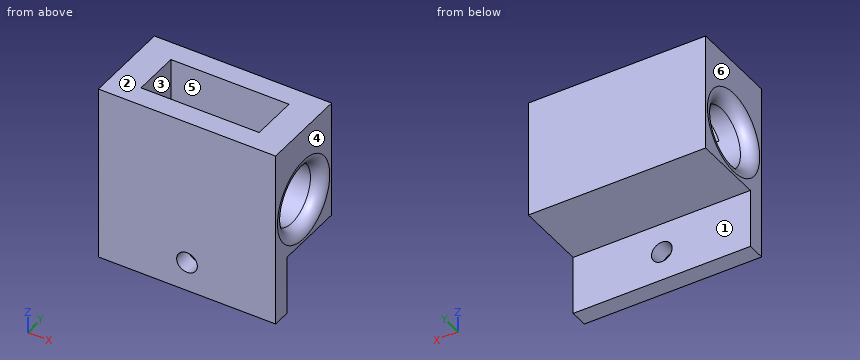
Autodesk Inventor part; units mm, degrees
ref_plane "YZ Plane" through (0, 0, 0) normal (1, 0, 0) x (0, 1, 0)
ref_plane "XZ Plane" through (0, 0, 0) normal (0, 1, 0) x (-1, 0, 0)
ref_plane "XY Plane" through (0, 0, 0) normal (0, 0, 1) x (1, 0, 0)
sketch "Esquisse1" plane through (0, 0, 0) normal (1, 0, 0) x (0, 1, 0)
  circle A0 centre (0, 0) radius 5
  line L0 (7.5, 7.5) -> (-7.5, 7.5)
  line L1 (-7.5, 7.5) -> (-7.5, -7.5)
  line L2 (-7.5, -7.5) -> (7.5, -7.5)
  line L3 (7.5, -7.5) -> (7.5, 7.5)
  line L4 (7.5, 7.5) -> (-7.5, -7.5)
  line L5 (-7.5, 7.5) -> (7.5, -7.5)
  point P0 (0, 0)
  dimension "d0" = 10
  dimension "d1" = 15
  dimension "d2" = 15
extrude "Extrusion1" add sketch "Esquisse1" along normal blind 30 contours A0 L4 L3 L5 | A0 L5 L0 L4 | L5 L2 L4 A0 | A0 L4 L1 L5
sketch "Esquisse6" plane through (0, -7.5, 7.5) normal (0, 0, 1) x (1, 0, 0)
  line L0 (0, 7.5) -> (30, 7.5)
  line L1 (30, 15) -> (30, 0)
  line L2 (5, 11.5) -> (25, 11.5)
  line L3 (25, 11.5) -> (25, 7.5)
  line L4 (25, 7.5) -> (5, 7.5)
  line L5 (5, 7.5) -> (5, 11.5)
  line L6 (0, 15) -> (0, 0)
  line L7 (0, 11.5) -> (5, 11.5)
  line L8 (5, 3.5) -> (25, 3.5)
  line L9 (25, 3.5) -> (25, 7.5)
  line L10 (5, 7.5) -> (5, 3.5)
  dimension "d14" = 4
  dimension "d15" = 5
  dimension "d16" = 20
extrude "Extrusion5" cut sketch "Esquisse6" against normal blind 5 contours L5 L2 L3 L0 | L0 L9 L8 L10
sketch "Esquisse8" plane through (0, -7.5, 7.5) normal (0, 0, 1) x (1, 0, 0)
  line L0 (5, 11.5) -> (25, 11.5)
  line L1 (25, 3.5) -> (5, 3.5)
  line L2 (5, 11.5) -> (25, 11.5)
  line L3 (25, 11.5) -> (25, 3.5)
  line L4 (25, 3.5) -> (5, 3.5)
  line L5 (5, 3.5) -> (5, 11.5)
  line L6 (0, 15) -> (30, 15)
  line L7 (30, 15) -> (30, 0)
  line L8 (0, 15) -> (30, 15)
  line L9 (30, 15) -> (30, 0)
  line L10 (30, 0) -> (0, 0)
  line L11 (0, 0) -> (0, 15)
  point P0 (0, 7.5)
extrude "Extrusion6" add sketch "Esquisse8" along normal blind 5
sketch "Esquisse9" plane through (0, -7.5, -7.5) normal (0, 0, -1) x (-1, 0, 0)
  line L0 (0, 0) -> (-30, 0)
  line L1 (-30, 0) -> (0, 0)
  line L2 (0, 0) -> (0, 3)
  line L3 (0, 3) -> (-30, 3)
  line L4 (-30, 3) -> (-30, 0)
  point P0 (0, 7.5)
extrude "Extrusion7" add sketch "Esquisse9" along normal blind 10
sketch "Esquisse10" plane through (0, -4.5, -7.5) normal (0, 1, 0) x (1, 0, 0)
  circle A0 centre (15, 5) radius 1.75
  line L0 (0, 10) -> (30, 10)
  line L1 (30, 0) -> (30, 10)
  point P0 (0, -7.5)
  dimension "d23" = 3.5
  dimension "d24" = 5
  dimension "d25" = 15
extrude "Extrusion8" cut sketch "Esquisse10" against normal blind 10
fillet "Congé2" radius 2 2 edges at (0, -5, 0) (30, -5, 0)
properties part number "Pièce1_Impression 3D"
Input: part model. Units: mm. Frame: model coordinates. Face numbers are marked on the shaded views. A direction names the side the tool comes from. Coordinates: 2 decimals unless noted, no trailing zeros. Order: outer loops, then holes, each group sorted by start corner. A loop starts at its lowest first (then second) coordinate and runs counter-clockwise, first axis right, second up. Notation, with made-up numbers: M 45,-27 L 80,-27 A22 ccw 80,-11 Z; hole C 51.25,8.25 d2. An arc over 180 degrees is marked long. Answer in a Markdown table with one row per item.
(1) Section query D-D, the plane x = 15. Output: boundary loops of the cut face in (y, z), plus the area to 3 significant figures.
Numbers:
| item | result |
|---|---|
| outline | M -7.5,-17.5 L -4.5,-17.5 L -4.5,-14.25 L -7.5,-14.25 Z; M -7.5,-10.75 L -4.5,-10.75 L -4.5,-7.5 L 7.5,-7.5 L 7.5,12.5 L 4,12.5 L 4,3 A5 cw long -4,3 L -4,12.5 L -7.5,12.5 Z |
| area | 176 mm^2 |
(2) Draft query along X for the marked faces 4, 5 and 6. Return one class per face: pulls with the +X half, pulls with the -X half, needs draft (parallel to the pull), parting line crosses it, or undercut.
Numbers:
| item | result |
|---|---|
| face 4 | pulls with the +X half |
| face 5 | undercut |
| face 6 | pulls with the -X half |
(3) Contact query for flat-ended pins moving along their axis: pin 1 Ø5 at (x, z) = (15.5, -10.5) entering from +Y; pin 2 Ø5 at (y, z) = (-3, 2.5) entering from -X; pin 3 Ø1.5 at (x, y) = (6.5, 5.5) entering from -Z. Output: stop coordinate, or through.
Numbers:
| item | result |
|---|---|
| pin 1 | stops at y = -4.5 |
| pin 2 | stops at x = 0.09 |
| pin 3 | stops at z = -7.5 |
(4) Section query A-A, the plane z = -12.5. Output: boundary loops of the cut face in (x, y), plus the area to 3 significant figures.
Numbers:
| item | result |
|---|---|
| outline | M 0,-7.5 L 13.25,-7.5 L 13.25,-4.5 L 0,-4.5 Z; M 16.75,-7.5 L 30,-7.5 L 30,-4.5 L 16.75,-4.5 Z |
| area | 79.5 mm^2 |
(5) Material intervals for line 1 (Z direction, x = 15, y = -5.9); line 2 (Y direction, x = 16, z = 0); line 3 (X direction, y = 1.75, z = 10.5), sorted ascending. Write a range as [from, to].
Numbers:
| item | result |
|---|---|
| line 1 | z = [-17.5, -14.25], [-10.75, 12.5] |
| line 2 | y = [-7.5, -5], [5, 7.5] |
| line 3 | x = [0, 5], [25, 30] |
(6) Access query for the marked faces 1, 2 and 3. Directions: +Z, -Z, +X, -X, +Y, -Y. A direction counts if a zero-diameter tool reaches every point of the face in a straight line with its end or side. Return the directions, or none.
Numbers:
| item | result |
|---|---|
| face 1 | -Z, +X, -X, +Y |
| face 2 | +Z, +X, -X, +Y, -Y |
| face 3 | +Z |
(7) Section query C-C, the plane y = 0. Output: boundary loops of the cut face in (x, z), plus the area to 3 significant figures.
Numbers:
| item | result |
|---|---|
| outline | M 0,-7.5 L 30,-7.5 L 30,-7 A2 ccw 28,-5 L 2,-5 A2 ccw 0,-7 Z; M 0,7 A2 ccw 2,5 L 5,5 L 5,12.5 L 0,12.5 Z; M 25,5 L 28,5 A2 ccw 30,7 L 30,12.5 L 25,12.5 Z |
| area | 147 mm^2 |
(8) Section query B-B, the plane x = 26. Output: boundary loops of the cut face in (y, z), plus the area to 3 significant figures.
Numbers:
| item | result |
|---|---|
| outline | M -7.5,-17.5 L -4.5,-17.5 L -4.5,-7.5 L 7.5,-7.5 L 7.5,12.5 L -7.5,12.5 Z; hole C 0,0 d10 |
| area | 251 mm^2 |
